Verification items for the finished model (mm, model axes). Face numbers are marked on the shaded views. A direction names the side the tool comes from. Give positions to 0.01 mm unless a question says otherwise; leave off trailing zeros. Order: outer loops, then holes, each group sorted by start corner. A loop starts at its lowest first (then second) coordinate and runs counter-clockwise, first axis right, second up. Notation, with made-up numbers: (67, 81) -> (85, 81) arc R17 ccw to (85, 113) -> close; hole circle Ø4 at (53, 5.25). An arc over 180 degrees is marked (long way). Write each question's results on one line, items separated by ' | '. Start each with the question number.
1. Cross-section at D-D, the plane x = -42. Enter the section's corners in (y, z), then the cut area to 3 significant figures.
2. Material ranges on L1, parallel to Z at x = -0.5, y = 6; L2, parallel to X at y = 6.55, z = 0; L3, parallel to X at y = 4.6, z = 0, recorded low to high. Write a range as from..to.
3. Cross-section at B-B, the plane x = 28.25. Enter the section's corners in (y, z), then the cut area to 3 significant figures.
4. Cross-section at A-A, the plane z = 28.25. Enter the section's corners in (x, y), then the cut area to 3 significant figures.
5. Depth check by flat-ended pin: pin 1 Ø10.5 at (x, z) = (-13.44, -13.44) entering from -Y; pin 2 Ø9.5 at (x, z) = (48.93, 28.25) entering from +Y; pin 3 Ø3 at (x, y) = (42.5, 23.5) entering from +Z; pin 4 Ø5.5 at (x, z) = (-48.93, 28.25) entering from +Y. Enter the tip coordinate at first touch or a pass-through.
6. Mould release check, pull along Z, two halves, no side actions. Record for the marked faces 3, 4 and 5: +Z half, -Z half, draft (parallel to the pull), parting line (faces both ways), or undercut.
7. Cross-section at C-C, the plane y = 12. State how many separate pieces and enclosed holes the cut face has, then the cut area to 3 significant figures.
8. Set-up check for the marked faces 1 and 2: record each of +Z, -Z, +X, -X, +Y, -Y from which the full face is reachable in a straight line by a thin tool's end or side.
from build123d import *

# Parameters (mm, degrees)
SKETCH4_R           = 3
CUT_EXTRUDE1_DEPTH  = 10
SKETCH5_R           = 4
CUT_EXTRUDE2_DEPTH  = 10
SKETCH6_W           = 2
SKETCH6_H           = 3
BOSS_EXTRUDE1_DEPTH = 6


with BuildPart() as part:
    # Sketch1 → Revolve1 (revolve)
    with BuildSketch(Plane.XY):
        Polygon((10.5, 32.216109623), (10.5, 39.216109623), (48, 39.216109623), (48, 9.216109623), (7.5, 9.216109623), (7.5, 3.216109623), (10, 3.216109623), (10, 6.216109623), (36, 6.216109623), (36, 4.216109623), (39, 4.216109623), (39, 6.216109623), (62.5, 6.216109623), (62.5, 14.216109623), (51.5, 14.216109623), (51.5, 43.216109623), (7.5, 43.216109623), (7.5, 32.216109623), align=None)
    revolve(axis=Axis((0, 0, 0), (0, 1, 0)))

    # Sketch4 → Cut-Extrude1 (cut)
    with BuildSketch(Plane(origin=(0, 14.216109623, 0), x_dir=(1, 0, 0), z_dir=(0, 1, 0))):
        with Locations((56.5, 0)):
            Circle(SKETCH4_R)
        with Locations((48.930435314, -28.25)):
            Circle(SKETCH4_R)
        with Locations((28.25, -48.930435314)):
            Circle(SKETCH4_R)
        with Locations((0, -56.5)):
            Circle(SKETCH4_R)
        with Locations((-28.25, -48.930435314)):
            Circle(SKETCH4_R)
        with Locations((-48.930435314, -28.25)):
            Circle(SKETCH4_R)
        with Locations((-56.5, 0)):
            Circle(SKETCH4_R)
        with Locations((-48.930435314, 28.25)):
            Circle(SKETCH4_R)
        with Locations((-28.25, 48.930435314)):
            Circle(SKETCH4_R)
        with Locations((0, 56.5)):
            Circle(SKETCH4_R)
        with Locations((28.25, 48.930435314)):
            Circle(SKETCH4_R)
        with Locations((48.930435314, 28.25)):
            Circle(SKETCH4_R)
    extrude(amount=-CUT_EXTRUDE1_DEPTH, mode=Mode.SUBTRACT)

    # Sketch5 → Cut-Extrude2 (cut)
    with BuildSketch(Plane(origin=(0, 43.216109623, 0), x_dir=(1, 0, 0), z_dir=(0, 1, 0))):
        with Locations((19, 0)):
            Circle(SKETCH5_R)
        with Locations((13.435028843, -13.435028843)):
            Circle(SKETCH5_R)
        with Locations((0, -19)):
            Circle(SKETCH5_R)
        with Locations((-13.435028843, -13.435028843)):
            Circle(SKETCH5_R)
        with Locations((-19, 0)):
            Circle(SKETCH5_R)
        with Locations((-13.435028843, 13.435028843)):
            Circle(SKETCH5_R)
        with Locations((0, 19)):
            Circle(SKETCH5_R)
        with Locations((13.435028843, 13.435028843)):
            Circle(SKETCH5_R)
    extrude(amount=-CUT_EXTRUDE2_DEPTH, mode=Mode.SUBTRACT)

    # Sketch6 → Boss-Extrude1 (add)
    with BuildSketch(Plane.XZ.offset(-3.216109623)):
        with Locations((0, 7.5)):
            Rectangle(SKETCH6_W, SKETCH6_H)
    extrude(amount=-BOSS_EXTRUDE1_DEPTH)


solid = part.part
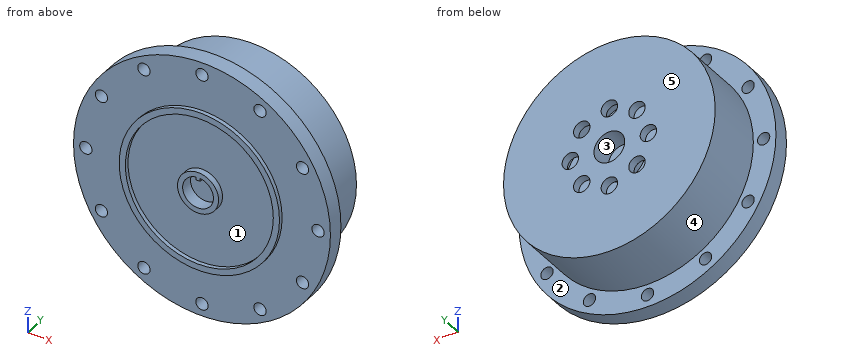
Results below:
1) outline: (6.22, -46.28) -> (14.22, -46.28) -> (14.22, -29.8) -> (43.22, -29.8) -> (43.22, 29.8) -> (14.22, 29.8) -> (14.22, 46.28) -> (6.22, 46.28) -> close; hole (9.22, -23.24) -> (39.22, -23.24) -> (39.22, 23.24) -> (9.22, 23.24) -> close | area: 1,070 mm²
2) L1: z = -39..-36, -9.99..-7.48, 6..9.99, 36..39 | L2: x = -62.5..-59.5, -53.5..-7.5, 7.5..53.5, 59.5..62.5 | L3: x = -39..-36, -10..-7.5, 7.5..10, 36..39
3) outline: (4.22, -26.89) -> (6.22, -26.89) -> (6.22, -45.93) -> (14.22, -45.93) -> (14.22, -43.06) -> (43.22, -43.06) -> (43.22, 43.06) -> (14.22, 43.06) -> (14.22, 45.93) -> (6.22, 45.93) -> (6.22, 26.89) -> (4.22, 26.89) -> (4.22, 22.31) -> (6.22, 22.31) -> (6.22, -22.31) -> (4.22, -22.31) -> close; (6.22, -55.75) -> (14.22, -55.75) -> (14.22, -51.93) -> (6.22, -51.93) -> close; (6.22, 51.93) -> (14.22, 51.93) -> (14.22, 55.75) -> (6.22, 55.75) -> close; hole (9.22, -38.81) -> (39.22, -38.81) -> (39.22, 38.81) -> (9.22, 38.81) -> close | area: 983 mm²
4) outline: (-55.75, 6.22) -> (-51.93, 6.22) -> (-51.93, 14.22) -> (-55.75, 14.22) -> close; (-45.93, 6.22) -> (-26.89, 6.22) -> (-26.89, 4.22) -> (-22.31, 4.22) -> (-22.31, 6.22) -> (22.31, 6.22) -> (22.31, 4.22) -> (26.89, 4.22) -> (26.89, 6.22) -> (45.93, 6.22) -> (45.93, 14.22) -> (43.06, 14.22) -> (43.06, 43.22) -> (-43.06, 43.22) -> (-43.06, 14.22) -> (-45.93, 14.22) -> close; (51.93, 6.22) -> (55.75, 6.22) -> (55.75, 14.22) -> (51.93, 14.22) -> close; hole (-38.81, 9.22) -> (38.81, 9.22) -> (38.81, 39.22) -> (-38.81, 39.22) -> close | area: 983 mm²
5) pin 1: stops at y = 6.22 | pin 2: stops at y = 14.22 | pin 3: stops at z = 31.16 | pin 4: passes through
6) face 3: undercut | face 4: parting line | face 5: draft
7) separate pieces: 1 | enclosed holes: 13 | area: 4,690 mm²
8) face 1: -Y | face 2: +Y
